from build123d import *

# Parameters (mm, degrees)
F2_DEPTH = 7


with BuildPart() as f2:
    # F1 (on Top) → F2 (new body)
    with BuildSketch(Plane.XY):
        with BuildLine():
            ThreePointArc((14, 0), (0, -14), (-14, 0))
            ThreePointArc((-14, 0), (-17.5, 3.5), (-21, 0))
            ThreePointArc((-21, 0), (0, -21), (21, 0))
            Line((21, 0), (21, 80))
            Line((21, 80), (150.3, 80))
            Line((150.3, 80), (150.3, 0))
            Line((150.3, 0), (155.3, 0))
            ThreePointArc((155.3, 0), (156.7142135624, 0.5857864376), (157.3, 2))
            Line((157.3, 2), (157.3, 85))
            ThreePointArc((157.3, 85), (156.7142135624, 86.4142135624), (155.3, 87))
            Line((155.3, 87), (16, 87))
            ThreePointArc((16, 87), (14.5857864376, 86.4142135624), (14, 85))
            Line((14, 85), (14, 0))
        make_face()
    extrude(amount=F2_DEPTH)


solid = f2.part
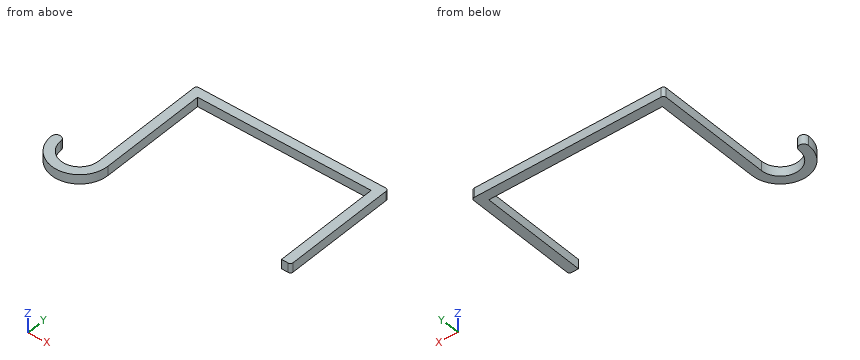
The listing builds one solid part. Answer for the finished solid, in the listing's coordinates (mm). Give positions to 0.01 mm unless a question says otherwise; leave off trailing zeros. Loops run counter-clockwise (first coordinate to the right, second up) from the corner with the lowest first, then second, coordinate; pieces in that order, holes last. Notation, with made-up numbers: (4, 64.5) - (13, 64.5) arc R31 ccw to (13, 101.5) - close; hole circle Ø3 at (-6, 70). An arc over 180 degrees is marked (long way). Use one line per item in the form item = value.
1. Find the intervals of material crossed by line 1 along X through (y, z) = (29, 1); line 2 along Y through (x, z) = (150, 4); line 3 along Y through (x, z) = (8, 1.5), in increasing order. Write a range as [from, to].
Calculated:
line_1 = [14, 21], [150.3, 157.3]
line_2 = [80, 87]
line_3 = [-19.42, -11.49]
2. Section D-D on x = -17.5 is taken. Give the vertices of the cut face in (y, z), then the cut area to 3 significant figures.
Calculated:
outline = (-11.61, 0) - (3.5, 0) - (3.5, 7) - (-11.61, 7) - close
area = 106 mm^2
3. Section A-A on y = 29 is taken. Give the vertices of the cut face in (x, z).
Calculated:
outline = (14, 0) - (21, 0) - (21, 7) - (14, 7) - close; (150.3, 0) - (157.3, 0) - (157.3, 7) - (150.3, 7) - close
4. Given pin 1 Ø3.5 at (y, z) = (51, 2) entering from -X; pin 2 Ø3 at (x, z) = (88, 5.5) entering from -Y; pin 3 Ø1.5 at (y, z) = (2.5, 1.5) entering from -X, each flat-ended and moving along its own axis, determine where each tip first touches the part or whether it passes through.
Calculated:
pin_1 = 14
pin_2 = 80
pin_3 = -20.53
5. Section B-B on z = 5 is taken. Give the vertices of the cut face in (x, y), then the cut area to 3 significant figures.
Calculated:
outline = (-21, 0) arc R21 ccw to (21, 0) - (21, 80) - (150.3, 80) - (150.3, 0) - (155.3, 0) arc R2 ccw to (157.3, 2) - (157.3, 85) arc R2 ccw to (155.3, 87) - (16, 87) arc R2 ccw to (14, 85) - (14, 0) arc R14 cw to (-14, 0) arc R3.5 ccw to start
area = 2,520 mm^2
6. Section C-C on x = 145 is taken. Give the vertices of the cut face in (y, z).
Calculated:
outline = (80, 0) - (87, 0) - (87, 7) - (80, 7) - close
